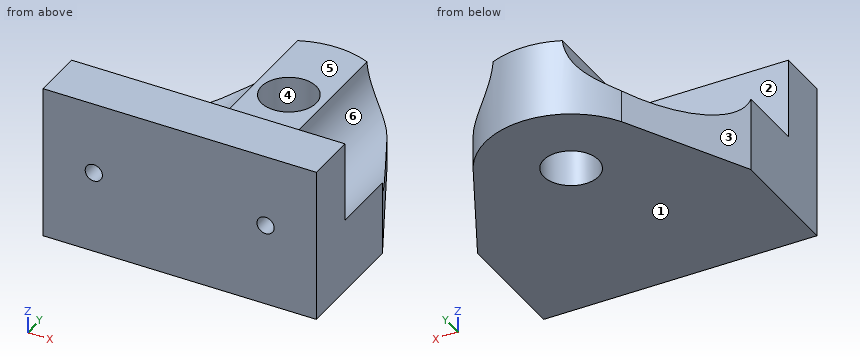
Autodesk Inventor part; units mm, degrees
ref_plane "YZ Plane" through (0, 0, 0) normal (1, 0, 0) x (0, 1, 0)
ref_plane "XZ Plane" through (0, 0, 0) normal (0, 1, 0) x (-1, 0, 0)
ref_plane "XY Plane" through (0, 0, 0) normal (0, 0, 1) x (1, 0, 0)
sketch "Sketch1" plane through (0, 0, 0) normal (0, 0, 1) x (1, 0, 0)
  circle A0 centre (10, 11.5) radius 1.6
  line L0 (0, 0) -> (20.0001, 0)
  line L1 (0, 0) -> (0, 3)
  line L2 (20.0001, 0) -> (20.0001, 3)
  line L3 (0, 3) -> (16, 3) construction
  line L4 (20.0001, 3) -> (36.0001, 3) construction
  arc A1 (14.3301, 14) -> (5.6699, 14) centre (10, 11.5) ccw
  line L5 (10, 11.5) -> (5.6699, 14) construction
  line L6 (10, 11.5) -> (14.3301, 14) construction
  line L7 (5.6699, 14) -> (0, 3)
  line L8 (14.3301, 14) -> (20.0001, 3)
  dimension "d17" = 3
  dimension "d18" = 3
  dimension "d19" = 11.5
  dimension "d23" = 90
  dimension "d24" = 90
  dimension "d25" = 10
  dimension "d31" = 5
  dimension "d32" = 120
  dimension "d33" = 14
extrude "Extrusion1" add sketch "Sketch1" along normal blind 4.5
sketch "Sketch4" plane through (0, 0, 4.5) normal (0, 0, 1) x (1, 0, 0)
  line L0 (0, 3) -> (0, 0)
  line L1 (20.0001, 0) -> (20.0001, 3)
  line L2 (0, 0) -> (20.0001, 0)
  line L3 (20.0001, 0) -> (20.0001, 3)
  line L4 (3.884, 22.9404) -> (-0.9789, 3.2417)
  line L5 (20.0001, 3) -> (0, 3)
  line L6 (0, 3) -> (0, 0)
extrude "Extrusion2" add sketch "Sketch4" along normal blind 4.5
sketch "Sketch5" plane through (0, 0, 0) normal (0, -1, 0) x (1, 0, 0)
  circle A0 centre (5, 4.8) radius 0.5
  circle A1 centre (15, 4.8) radius 0.5
  line L0 (0, 0) -> (20.0001, 0)
  dimension "d13" = 1
  dimension "d14" = 1
  dimension "d38" = 4.8
  dimension "d39" = 4.8
extrude "Extrusion3" cut sketch "Sketch5" against normal through all
sketch "Sketch6" plane through (0, 3, 9) normal (0, 1, 0) x (1, 0, 0)
  circle A0 centre (5, 4.2) radius 0.5
  circle A1 centre (5, 4.2) radius 3
  circle A2 centre (15, 4.2) radius 0.5
  circle A3 centre (15, 4.2) radius 3
  line L0 (0, 9) -> (20.0001, 9)
  dimension "d34" = 6
  dimension "d35" = 6
  dimension "d40" = 4.8
  dimension "d41" = 4.8
extrude "Extrusion4" cut sketch "Sketch6" along normal up to next
sketch "Sketch7" plane through (0, 0, 0) normal (0, -1, 0) x (1, 0, 0)
  line L0 (0, 0) -> (0, 9)
  line L1 (2.042, 0) -> (0, 0)
  line L2 (0, 0) -> (0, 9)
  line L3 (0, 9) -> (2.042, 9)
  line L4 (2.042, 9) -> (2.042, 0)
extrude "Extrusion5" cut sketch "Sketch7" against normal up to next
sketch "Sketch8" plane through (20.0001, 0, 0) normal (0, -1, 0) x (1, 0, 0)
  line L0 (0, 4.5) -> (0, 9)
  line L1 (-2.042, 0) -> (0, 0)
  line L2 (0, 0) -> (0, 9)
  line L3 (0, 9) -> (-2.042, 9)
  line L4 (-2.042, 9) -> (-2.042, 0)
  point P0 (-20.0001, 0)
extrude "Extrusion6" cut sketch "Sketch8" against normal up to next
properties part number "lower_deck_shaft_mount_printing_org"
The model under review builds one solid part; all positions refer to its coordinate system, in mm. Face numbers are marked on the shaded views. A direction names the side the tool comes from. Give positions to 0.01 mm unless a question says otherwise; leave off trailing zeros. Loops run counter-clockwise (first coordinate to the right, second up) from the corner with the lowest first, then second, coordinate; pieces in that order, holes last. Notation, with made-up numbers: (86, 31) -> (100, 31) arc R11 cw to (100, 43) -> close; hole circle Ø3 at (68, 25.5). An arc over 180 degrees is marked (long way). Write each question's results on one line, items separated by ' | '.
1) Take a section at B-B, the plane x = 10. Give the boundary of the cut face in (y, z), plus the area to 4 significant figures.
Conclusion:
outline: (0, 0) -> (9.9, 0) -> (9.9, 4.5) -> (3, 4.5) -> (3, 9) -> (0, 9) -> close; (13.1, 0) -> (16.5, 0) -> (16.5, 4.5) -> (13.1, 4.5) -> close | area: 73.35 mm^2
2) Tool access review of the marked faces 4, 5 and 6: name each direction out of +Z, -Z, +X, -X, +Y, -Y from which nothing blocks a thin tool from reaching the whole face with its end or side.
Conclusion:
face 4: +Z, -Z | face 5: +Z, +X, -X, +Y | face 6: +Z, +Y
3) Take a section at C-C, the plane y = 11. Give the boundary of the cut face in (x, z), plus the area to 3 significant figures.
Conclusion:
outline: (4.12, 0) -> (8.48, 0) -> (8.48, 4.5) -> (7.98, 4.5) arc R3 cw to (4.12, 1.93) -> close; (11.52, 0) -> (15.88, 0) -> (15.88, 1.93) arc R3 cw to (12.02, 4.5) -> (11.52, 4.5) -> close | area: 22.2 mm^2
4) Take a section at A-A, the plane z = 4.8. Give the boundary of the cut face in (x, y), plus the area to 3 significant figures.
Conclusion:
outline: (2.04, 0) -> (4.5, 0) -> (4.5, 3) -> (2.04, 3) -> close; (5.5, 0) -> (14.5, 0) -> (14.5, 3) -> (5.5, 3) -> close; (15.5, 0) -> (17.96, 0) -> (17.96, 3) -> (15.5, 3) -> close | area: 41.7 mm^2
5) For line 1 along Z through (x, y) = (15, 1.6); line 2 along Y through (x, z) = (9.5, 0.5); line 3 along Y through (x, z) = (13.5, 3), list the stretches that pass through material, from the lowest coordinate up. Write a range as from..to.
Conclusion:
line 1: z = 0..4.3, 5.3..9 | line 2: y = 0..9.98, 13.02..16.47 | line 3: y = 0..3
6) Insertion check: pin 1 Ø2 at (y, z) = (11.5, 1) entering from +X; pin 2 Ø3 at (x, y) = (7.5, 8.5) entering from +Z. Each pin has a flat end and moves straight along its axis. Give the tip position at first contact, or say it passes through.
Conclusion:
pin 1: stops at x = 16.13 | pin 2: stops at z = 4.5
7) Take a section at D-D, the plane z = 3.5. Give the boundary of the cut face in (x, y), plus the area to 3 significant figures.
Conclusion:
outline: (2.04, 0) -> (17.96, 0) -> (17.96, 6.96) -> (17.7, 7.46) -> (17.7, 3) -> (12.3, 3) -> (12.3, 15.94) arc R5 ccw to (7.7, 15.94) -> (7.7, 3) -> (2.3, 3) -> (2.3, 7.45) -> (2.04, 6.96) -> close; hole circle Ø3.2 at (10, 11.5) | area: 103 mm^2
8) Draft analysis for pull direction X (two halves, no side actions). For the marked faces 1, 2 and 3, state which applies: pulls with the +X half, pulls with the -X half, needs draft (parallel to the pull), parting line crosses it, or undercut.
Conclusion:
face 1: needs draft | face 2: undercut | face 3: pulls with the -X half
